Build history of the part. All positions in model axes, mm. A direction names the side the tool comes from. Round coordinates to 2 decimals unless told otherwise and drop trailing zeros. Write each loop counter-clockwise with the first axis right and the second up, starting at its lowest first coordinate (ties: lowest second). Pieces come first, ordered by that corner, then holes. Notation, with made-up numbers: (45.5, 17.25) -> (95.5, 17.25) arc R32 ccw to (95.5, 50.25) -> close; hole circle Ø11 at (-12, 67.25). An arc over 180 degrees is marked (long way). Answer in a Markdown table with one row per item.
Autodesk Inventor part; units mm, degrees
ref_plane "YZ Plane" through (0, 0, 0) normal (1, 0, 0) x (0, 1, 0)
ref_plane "XZ Plane" through (0, 0, 0) normal (0, 1, 0) x (-1, 0, 0)
ref_plane "XY Plane" through (0, 0, 0) normal (0, 0, 1) x (1, 0, 0)
sketch "Sketch1" plane through (0, 0, 0) normal (1, 0, 0) x (0, 1, 0)
  circle A0 centre (0, 0) radius 6.35
  dimension "d0" = 12.7
extrude "Extrusion1" add sketch "Sketch1" along normal blind 127
sketch "Sketch2" plane through (127, 0, 0) normal (1, 0, 0) x (0, 0, -1)
  circle A0 centre (0, 0) radius 46.74
extrude "Extrusion2" cut sketch "Sketch2" against normal blind 6.35
sketch "Sketch3" plane through (120.65, 0, 0) normal (1, 0, 0) x (0, 0, -1)
  arc A0 (0, 0) -> (23.8252, 33.0958) centre (-7.3529, 30.4168) ccw
  arc A1 (23.8252, 33.0958) -> (0, 0) centre (27.6846, 5.1939) ccw
extrude "Extrusion3" add sketch "Sketch3" against normal blind 4.7625
pattern_circular "Circular Pattern1" count 3 over 360 about axis through (0, 0, 0) along (1, 0, 0) of "Extrusion3"
properties part number "Motor Axle"
Q1. Saw through at C-C on x = 107.5. Write the cut outline in (y, z), plus the area to 3 significant figures.
A:
| item | result |
|---|---|
| outline | circle Ø12.7 at (0, 0) |
| area | 127 mm² |
Q2. Two-plate mould, pull along Y, no slides. Class faces 1 (the flat face through (0, 0, 0)), 2 (the cylindrical face through (118.3, -6.09, 24.57)), 3 (the cylindrical face through (118.3, 14.57, -19.63)), 4 (the cylindrical face through (118.3, -18.23, -17.56)): released by +Y, released by -Y, zero draft, split by the parting line, or undercut.
A:
| item | result |
|---|---|
| face 1 | zero draft |
| face 2 | released by -Y |
| face 3 | undercut |
| face 4 | undercut |
Q3. Saw through at B-B on z = -2. Write the cut outline in (x, y).
A:
| item | result |
|---|---|
| outline | (0, -6.03) -> (115.89, -6.03) -> (115.89, -22.78) -> (120.65, -22.78) -> (120.65, 16.76) -> (115.89, 16.76) -> (115.89, 6.03) -> (0, 6.03) -> close |
Q4. Drop flat-ended pins along their axis: P1, Ø12, axis at y = 17, z = 15, coming from the -X side; P2, Ø5, axis at y = -7, z = 26.5, coming from the +X side; P3, Ø1.5, axis at y = 9, z = -10, coming from the -X side; P4, Ø10, axis at x = 31, z = -9, coming from the -Y side. Give the stop position or say it passes through.
A:
| item | result |
|---|---|
| P1 | through |
| P2 | x = 120.65 |
| P3 | x = 115.89 |
| P4 | y = -4.93 |
Q5. Saw through at D-D on y = 0. Write the cut outline in (x, z).
A:
| item | result |
|---|---|
| outline | (0, -6.35) -> (120.65, -6.35) -> (120.65, 36.68) -> (115.89, 36.68) -> (115.89, 6.35) -> (0, 6.35) -> close |
Q6. Saw through at A-A on z = -13. Write the cut outline in (x, y), plus the area to 3 significant figures.
A:
| item | result |
|---|---|
| outline | (115.89, -35.1) -> (120.65, -35.1) -> (120.65, -9.42) -> (115.89, -9.42) -> close; (115.89, 6.65) -> (120.65, 6.65) -> (120.65, 29.23) -> (115.89, 29.23) -> close |
| area | 230 mm² |
Q7. Wall check: line 1 (X direction, y = -28, z = -13.5); line 2 (Y direction, x = 44.5, z = 4); line 3 (Y direction, x = 24, z = 1). Give the ranges that are in metal, low to high. Write a range as [from, to].
A:
| item | result |
|---|---|
| line 1 | [115.89, 120.65] |
| line 2 | [-4.93, 4.93] |
| line 3 | [-6.27, 6.27] |
Q8. Which spindle directions (+Z, -Z, +X, -X, +Y, -Y) get a long thin tool onto all of the face, cutting with end or side? Do faces 5 (the flat face through (120.65, -1, 0)), 6 (the cylindrical face through (59.48, -1.38, 6.2)). Say none if no direction does.
A:
| item | result |
|---|---|
| face 5 | +Z, -Z, +X, +Y, -Y |
| face 6 | -X |
